CAD build for the part. Positions are in the model's coordinates, mm. A direction names the side the tool comes from. Coordinates: 2 decimals unless noted, no trailing zeros. Write each loop counter-clockwise with the first axis right and the second up, starting at its lowest first coordinate (ties: lowest second). Pieces come first, ordered by that corner, then holes.
```python
from build123d import *

# Parameters (mm, degrees)
IZIM1_R                     = 1.388888889
Y_KSEKLIK_EKSTR_ZYON1_DEPTH = 10
IZIM2_R                     = 2.5
Y_KSEKLIK_EKSTR_ZYON2_DEPTH = 15


with BuildPart() as part:
    # Çizim1 → Yükseklik-Ekstrüzyon1 (new body)
    with BuildSketch(Plane.XY.offset(10)):
        with BuildLine():
            Line((11.575672227, 67.181181276), (4.575672227, 67.181181276))
            ThreePointArc((4.575672227, 67.181181276), (2.454351883, 66.30250162), (1.575672227, 64.181181276))
            Line((1.575672227, 64.181181276), (1.575672227, 4.181181276))
            ThreePointArc((1.575672227, 4.181181276), (7.433536603, -9.960954347), (21.575672227, -15.818818724))
            Line((21.575672227, -15.818818724), (31.075672227, -15.818818724))
            ThreePointArc((31.075672227, -15.818818724), (45.21780785, -9.960954347), (51.075672227, 4.181181276))
            Line((51.075672227, 4.181181276), (51.075672227, 64.181181276))
            ThreePointArc((51.075672227, 64.181181276), (50.19699257, 66.30250162), (48.075672227, 67.181181276))
            Line((48.075672227, 67.181181276), (41.075672227, 67.181181276))
            Line((41.075672227, 67.181181276), (41.075672227, 78.181181276))
            Line((41.075672227, 78.181181276), (11.575672227, 78.181181276))
            Line((11.575672227, 78.181181276), (11.575672227, 67.181181276))
        make_face()
        with Locations(Location((16.795672227, 72.222222222, 0), (0, 0, 180))):
            Circle(IZIM1_R, mode=Mode.SUBTRACT)
        with Locations(Location((35.853450004, 72.222222222, 0), (0, 0, 180))):
            Circle(IZIM1_R, mode=Mode.SUBTRACT)
    extrude(amount=-Y_KSEKLIK_EKSTR_ZYON1_DEPTH)

    # Çizim2 → Yükseklik-Ekstrüzyon2 (add)
    with BuildSketch(Plane.XY.offset(10)):
        with Locations((26.575672227, 1.181181276)):
            Circle(IZIM2_R)
    extrude(amount=Y_KSEKLIK_EKSTR_ZYON2_DEPTH)


solid = part.part
```
Item 1: Saw through at D-D, the plane x = 45. Write the cut outline in (y, z).
Item 2: Saw through at A-A, the plane x = 25.5. Write the cut outline in (y, z).
Item 3: Saw through at B-B, the plane y = 10.5. Write the cut outline in (x, z).
Item 4: Which spindle directions (+Z, -Z, +X, -X, +Y, -Y) get a long thin tool onto all of the face, cutting with end or side? Do faces 4 (the flat face through (45, 67.181, 5)), 5 (the cylindrical face through (24.08, 1.29, 17.4)), 6 (the flat face through (11.576, 73, 5)). Say none if no direction does.
Item 5: Flat gauge pins, fed straight in: pin 1 Ø2 at (x, z) = (7.5, 5.5) entering from +Y; pin 2 Ø5 at (y, z) = (73, 7) entering from -X; pin 3 Ø3 at (y, z) = (72.5, 6) entering from +X; pin 4 Ø2.5 at (x, y) = (16.8, 72.22) entering from -Z. Where does each tip first touch, or does it go through?
Item 6: Saw through at C-C, the plane z = 11.5. Write the cut outline in (x, y).
Item 7: Wall check: line 1 along Z through (x, y) = (47, 28.5); line 2 along Y through (x, z) = (35.5, 8.25); line 3 along Y through (x, z) = (10.5, 2.5). Give the ranges that are in metal, low to high.
Item 8: Two-plate mould, pull along Y, no slides. Class faces 1 (the flat face through (8, 67.181, 5)), 2 (the cylindrical face through (16.976, 70.845, 5.07)), 3 (the flat face through (51.076, 34, 5)): +Y half, -Y half, draft (parallel to the pull), parting line (faces both ways), or undercut.
Working result:
1. outline: (-10.18, 0) - (67.18, 0) - (67.18, 10) - (-10.18, 10) - close
2. outline: (-15.82, 0) - (78.18, 0) - (78.18, 10) - (3.44, 10) - (3.44, 25) - (-1.08, 25) - (-1.08, 10) - (-15.82, 10) - close
3. outline: (1.58, 0) - (51.08, 0) - (51.08, 10) - (1.58, 10) - close
4. face 4: +Z, -Z, +X, +Y
4. face 5: +Z
4. face 6: +Z, -Z, -X, +Y
5. pin 1: stops at y = 67.18
5. pin 2: stops at x = 11.58
5. pin 3: stops at x = 41.08
5. pin 4: passes through
6. outline: circle Ø5 at (26.58, 1.18)
7. line 1: z = 0 to 10
7. line 2: y = -15.32 to 70.88, 73.57 to 78.18
7. line 3: y = -12.47 to 67.18
8. face 1: +Y half
8. face 2: undercut
8. face 3: draft
